Can you work these out from the model? Positions are in its coordinate system, mm. A direction names the side the tool comes from. Give positions to 0.01 mm unless a question says otherwise; leave off trailing zeros. Write each loop counter-clockwise with the first axis right and the second up, starting at its lowest first coordinate (ties: lowest second). Pieces come first, ordered by that corner, then holes. Notation, with made-up numbers: M 68,23.5 L 87,23.5 A24 ccw 87,55.5 Z; hole C 54,88 d10. An arc over 180 degrees is marked long. Write each question's results on one line, items separated by ' | '.
from build123d import *
from OCP.BRepFilletAPI import BRepFilletAPI_MakeFillet

# Parameters (mm, degrees)
SKETCH_1_W               = 20
SKETCH_1_H               = 32
SKETCH_1_R               = 1.35
EXTRUDE_1_DEPTH          = 2
EXTRUDE_2_DEPTH          = 2
FILLET_1_R               = 20
CUT_EXTRUDE_2_DEPTH      = 58.314919524
CUT_EXTRUDE_2_DEPTH_BACK = 58.314919524
FILLET_2_R1              = 2
FILLET_2_R2              = 1
FILLET_5_R               = 2
FILLET_6_R               = 30


with BuildPart() as part:
    # 草图1 → 凸台-拉伸1 (new body)
    with BuildSketch(Plane(origin=(0, 0, 0), x_dir=(1, 0, 0), z_dir=(0, 1, 0))):
        with Locations((0, -4)):
            Rectangle(SKETCH_1_W, SKETCH_1_H)
        with Locations(Location((-6, 10, 0), (0, 0, 270))):
            Circle(SKETCH_1_R, mode=Mode.SUBTRACT)
        with Locations(Location((6, 10, 0), (0, 0, 90))):
            Circle(SKETCH_1_R, mode=Mode.SUBTRACT)
        with Locations(Location((6, -10, 0), (0, 0, 270))):
            Circle(SKETCH_1_R, mode=Mode.SUBTRACT)
        with Locations(Location((-6, -10, 0), (0, 0, 90))):
            Circle(SKETCH_1_R, mode=Mode.SUBTRACT)
    extrude(amount=EXTRUDE_1_DEPTH)

    # 草图2 → 凸台-拉伸2 (add)
    with BuildSketch(Plane(origin=(0, 2, 0), x_dir=(1, 0, 0), z_dir=(0, 1, 0))):
        with BuildLine():
            Line((-40, 41), (-40, 13))
            Line((-40, 13), (-10, 13))
            Line((-10, 13), (-10, 12))
            Line((-10, 12), (10, 12))
            ThreePointArc((10, 12), (-0.654211509, 32.690782604), (-22.393061845, 41))
            Line((-22.393061845, 41), (-40, 41))
        make_face()
    extrude(amount=-EXTRUDE_2_DEPTH)

    # 圆角1
    fillet_1_edges = [part.edges().sort_by_distance(p)[0] for p in [
        (-10, 1, -13),
    ]]
    fillet(fillet_1_edges, radius=FILLET_1_R)

    # 草图3 → 切除-拉伸2 (cut, two sides: drawn at the far end of the back side and taken through both)
    with BuildSketch(Plane(origin=(0, 2, 0), x_dir=(1, 0, 0), z_dir=(0, 1, 0)).offset(-CUT_EXTRUDE_2_DEPTH_BACK)):
        Polygon((-22.393061845, 36), (-35, 36), (-35, 18), align=None)
        with BuildLine():
            Line((-31.337370064, 18), (-30, 18))
            ThreePointArc((-30, 18), (-21.339745962, 16.452078799), (-13.751923191, 12))
            Line((-13.751923191, 12), (-21.0069112, 32.749676509))
            Line((-21.0069112, 32.749676509), (-31.337370064, 18))
        make_face()
        with BuildLine():
            Line((-10.235217527, 11.031539438), (-18.887076306, 35.776345445))
            ThreePointArc((-18.887076306, 35.776345445), (-12.511241297, 34.169724991), (-6.696576783, 31.100168357))
            Line((-6.696576783, 31.100168357), (-10.235217527, 11.031539438))
        make_face()
        with BuildLine():
            Line((-6.665518003, 14), (4.625979988, 14))
            ThreePointArc((4.625979988, 14), (1.508463055, 22.192897882), (-4.021593898, 28.994438709))
            Line((-4.021593898, 28.994438709), (-6.665518003, 14))
        make_face()
    extrude(amount=CUT_EXTRUDE_2_DEPTH + CUT_EXTRUDE_2_DEPTH_BACK, mode=Mode.SUBTRACT)

    # 圆角2: one fillet with a radius per group of edges: ONE call of the kernel's fillet builder (fillet() takes one radius for all edges)
    fillet_2_edges_1 = [part.edges().sort_by_distance(p)[0] for p in [
        (-31.337370064, 1, -18),
        (-22.393061845, 1, -36),
        (-35, 1, -36),
        (-21.0069112, 1, -32.749676509),
        (-4.021593898, 1, -28.994438709),
        (-6.696576783, 1, -31.100168357),
        (-18.887076306, 1, -35.776345445),
        (4.625979988, 1, -14),
        (-6.665518003, 1, -14),
    ]]
    fillet_2_edges_2 = [part.edges().sort_by_distance(p)[0] for p in [
        (-35, 1, -18),
        (-13.751923191, 1, -12),
        (-10.235217527, 1, -11.031539438),
    ]]
    fillet_2 = BRepFilletAPI_MakeFillet(part.part.solid().wrapped)
    for e in fillet_2_edges_1:
        fillet_2.Add(FILLET_2_R1, e.wrapped)
    for e in fillet_2_edges_2:
        fillet_2.Add(FILLET_2_R2, e.wrapped)
    add(Compound.cast(fillet_2.Shape()), mode=Mode.REPLACE)

    # 圆角5
    fillet_5_edges = [part.edges().sort_by_distance(p)[0] for p in [
        (-40, 1, -13),
        (-40, 1, -41),
        (10, 1, 20),
        (-10, 1, 20),
    ]]
    fillet(fillet_5_edges, radius=FILLET_5_R)

    # 圆角6
    fillet_6_edges = [part.edges().sort_by_distance(p)[0] for p in [
        (10, 1, -12),
    ]]
    fillet(fillet_6_edges, radius=FILLET_6_R)


solid = part.part
Item 1: I want a section at A-A, the plane x = 6. Please give me the cut outline in (y, z), and give its area (3 significant figures).
Geometry says:
outline: M 0,-24.41 L 2,-24.41 L 2,-11.35 L 0,-11.35 Z; M 0,-8.65 L 2,-8.65 L 2,8.65 L 0,8.65 Z; M 0,11.35 L 2,11.35 L 2,20 L 0,20 Z | area: 78.0 mm2
Item 2: I want a section at C-C, the plane z = 6. Please give me the cut outline in (x, y), and give its area (4 significant figures).
Geometry says:
outline: M -10.03,0 L 10,0 L 10,2 L -10.03,2 Z | area: 40.05 mm2
Item 3: If I drill on line 1 (X direction, y = 1.5, z = 10); line 2 (X direction, y = 1.5, z = -10); line 3 (Z direction, x = -25, y = 0.75), over which ranges is the centre line in solid material (lowest first)? Write a range as from..to.
Geometry says:
line 1: x = -10..-7.35, -4.65..4.65, 7.35..10 | line 2: x = -19.46..-7.35, -4.65..4.65, 7.35..9.99 | line 3: z = -41..-35.57, -32.28..-27.05, -17.49..-12.36
Item 4: I'm going to push flat-ended pins straight in: pin 1 (1 mm diameter, centred on y = 1.5, z = 11.5, fed in from -X); pin 2 (0.6 mm diameter, centred on x = -29, y = 1, fed in from +Z). Where does each tip first touch, or does it pass through?
Geometry says:
pin 1: stops at x = -10 | pin 2: stops at z = -12.96
Item 5: I want a section at B-B, the plane y = 1. Give the number of separate pieces and of enclosed holes in the cut face, and give its area (3 significant figures).
Geometry says:
separate pieces: 1 | enclosed holes: 8 | area: 1,430 mm2
Item 6: Thinking about a two-plate mould opening in Z: for faces 4 (the face through (-39.43, 0.99, -40.4)), 5 (the face through (-15.703, 0.986, -6.986)), 6 (the face through (-5.594, 0.986, -8.712)), 7 (the face through (-17.338, 1.014, -34.485)), which applies, +Z half, -Z half, draft (parallel to the pull), parting line (faces both ways), or undercut?
Geometry says:
face 4: -Z half | face 5: +Z half | face 6: undercut | face 7: undercut
Item 7: For faces 1 (the face through (3.672, 1.014, -14.835)), 2 (the face through (-34, 1, -13)), 3 (the face through (-30, 1, -41)), which set-ups out of +Z, -Z, +X, -X, +Y, -Y let a thin tool reach every point of the face, with its end or its side?
Geometry says:
face 1: +Y, -Y | face 2: +Z, -X, +Y, -Y | face 3: -Z, +X, -X, +Y, -Y
